Verification items for the finished model (mm, model axes). A direction names the side the tool comes from. Round coordinates to 2 decimals unless told otherwise and drop trailing zeros. Write each loop counter-clockwise with the first axis right and the second up, starting at its lowest first coordinate (ties: lowest second). Pieces come first, ordered by that corner, then holes. Notation, with made-up numbers: M -34.75,22.5 L 2.25,22.5 A9 ccw 2.25,33.5 Z; hole C -35,28.5 d2. An arc over 180 degrees is marked long. Use a Markdown table: item, result. Add a question column.
from build123d import *

# Parameters (mm, degrees)
BOSS_EXTRUDE1_DEPTH = 7.5
SKETCH2_R           = 3.5
CUT_EXTRUDE1_DEPTH  = 44.649720503
SKETCH6_R           = 3.5
CUT_EXTRUDE4_DEPTH  = 52.358372248
CUT_EXTRUDE5_DEPTH  = 1
CUT_EXTRUDE6_DEPTH  = 53.041544942
CUT_EXTRUDE7_DEPTH  = 1
CUT_EXTRUDE8_DEPTH  = 44.649720503
BOSS_EXTRUDE2_DEPTH = 22
BOSS_EXTRUDE3_START = -40
SKETCH12_W          = 15
SKETCH12_H          = 5
BOSS_EXTRUDE3_DEPTH = 40
CUT_EXTRUDE9_DEPTH  = 5


with BuildPart() as part:
    # Sketch1 → Boss-Extrude1 (new, symmetric)
    with BuildSketch(Plane(origin=(0, 0, 0), x_dir=(0, 0, -1), z_dir=(1, 0, 0))):
        Polygon((-15.91, -3), (-15.91, 3), (15.91, 3), (15.91, 37), (21.91, 37), (21.91, -3), align=None)
    extrude(amount=BOSS_EXTRUDE1_DEPTH, both=True)

    # Sketch2 → Cut-Extrude1 (cut, through all)
    with BuildSketch(Plane(origin=(0, 0, 0), x_dir=(1, 0, 0), z_dir=(0, 1, 0))):
        with Locations(Location((0, -9.41, 0), (0, 0, 90))):
            Circle(SKETCH2_R)
    extrude(amount=CUT_EXTRUDE1_DEPTH, mode=Mode.SUBTRACT)

    # Sketch6 → Cut-Extrude4 (cut, through all)
    with BuildSketch(Plane.XY.offset(-18.91)):
        with Locations((0, 30.5)):
            Circle(SKETCH6_R)
    extrude(amount=-CUT_EXTRUDE4_DEPTH, mode=Mode.SUBTRACT)

    # Sketch7 → Cut-Extrude5 (cut, symmetric)
    with BuildSketch(Plane.XY.offset(-18.91)):
        with BuildLine():
            Line((2.235057553, 16.161122159), (3.84429899, 30.054730114))
            ThreePointArc((3.84429899, 30.054730114), (3.863569405, 30.276994499), (3.87, 30.5))
            Line((3.87, 30.5), (3.87, 37))
            Line((3.87, 37), (-3.87, 37))
            Line((-3.87, 37), (-3.87, 30.5))
            ThreePointArc((-3.87, 30.5), (-3.863569405, 30.276994499), (-3.84429899, 30.054730114))
            Line((-3.84429899, 30.054730114), (-2.235057553, 16.161122159))
            ThreePointArc((-2.235057553, 16.161122159), (0, 14.17), (2.235057553, 16.161122159))
        make_face()
    extrude(amount=CUT_EXTRUDE5_DEPTH, both=True, mode=Mode.SUBTRACT)

    # Sketch8 → Cut-Extrude6 (cut, through all)
    with BuildSketch(Plane.XY.offset(-19.91)):
        with BuildLine():
            Line((3.87, 30.5), (3.87, 37))
            Line((3.87, 37), (-3.87, 37))
            Line((-3.87, 37), (-3.87, 30.5))
            ThreePointArc((-3.87, 30.5), (0, 26.63), (3.87, 30.5))
        make_face()
    extrude(amount=CUT_EXTRUDE6_DEPTH, mode=Mode.SUBTRACT)

    # Sketch9 → Cut-Extrude7 (cut, symmetric)
    with BuildSketch(Plane(origin=(0, 0, 0), x_dir=(1, 0, 0), z_dir=(0, 1, 0))):
        with BuildLine():
            Line((-3.87, -9.41), (-3.87, -15.91))
            Line((-3.87, -15.91), (3.87, -15.91))
            Line((3.87, -15.91), (3.87, -9.41))
            ThreePointArc((3.87, -9.41), (3.863569405, -9.186994499), (3.84429899, -8.964730114))
            Line((3.84429899, -8.964730114), (2.235057553, 4.928877841))
            ThreePointArc((2.235057553, 4.928877841), (0, 6.92), (-2.235057553, 4.928877841))
            Line((-2.235057553, 4.928877841), (-3.84429899, -8.964730114))
            ThreePointArc((-3.84429899, -8.964730114), (-3.863569405, -9.186994499), (-3.87, -9.41))
        make_face()
    extrude(amount=CUT_EXTRUDE7_DEPTH, both=True, mode=Mode.SUBTRACT)

    # Sketch10 → Cut-Extrude8 (cut, through all)
    with BuildSketch(Plane(origin=(0, 0, 0), x_dir=(1, 0, 0), z_dir=(0, 1, 0))):
        with BuildLine():
            Line((-3.87, -15.91), (3.87, -15.91))
            Line((3.87, -15.91), (3.87, -9.41))
            ThreePointArc((3.87, -9.41), (0, -5.54), (-3.87, -9.41))
            Line((-3.87, -9.41), (-3.87, -15.91))
        make_face()
    extrude(amount=-CUT_EXTRUDE8_DEPTH, mode=Mode.SUBTRACT)

    # Sketch11 → Boss-Extrude2 (add)
    with BuildSketch(Plane.XY.offset(15.91)):
        Polygon((-7.5, -3), (-3.87, -3), (-3.87, 1), (3.87, 1), (3.87, -3), (7.5, -3), (7.5, 3), (-7.5, 3), align=None)
    extrude(amount=BOSS_EXTRUDE2_DEPTH)

    # Sketch12 → Boss-Extrude3 (add)
    with BuildSketch(Plane.XZ.offset(3).offset(BOSS_EXTRUDE3_START)):
        with Locations((0, 35.41)):
            Rectangle(SKETCH12_W, SKETCH12_H)
    extrude(amount=BOSS_EXTRUDE3_DEPTH)

    # Sketch14 → Cut-Extrude9 (cut)
    with BuildSketch(Plane.XY.offset(37.91)):
        with BuildLine():
            Line((-2.625, 37), (-2.625, 30.5))
            ThreePointArc((-2.625, 30.5), (0, 27.875), (2.625, 30.5))
            Line((2.625, 30.5), (2.625, 37))
            Line((2.625, 37), (-2.625, 37))
        make_face()
    extrude(amount=-CUT_EXTRUDE9_DEPTH, mode=Mode.SUBTRACT)


solid = part.part
1. Cross-section at D-D on z = 18.5. Enter the section's corners in (x, y).
2. Depth check by flat-ended pin: pin 1 Ø10 at (y, z) = (27, -10) entering from -X; pin 2 Ø6 at (y, z) = (9.5, -14) entering from -X; pin 3 Ø7.5 at (x, z) = (-2, 12.5) entering from +Y. Enter the tip coordinate at first touch or a pass-through.
3. Scan lines: line 1 along Z through (x, y) = (1.25, 23); line 2 along Z through (x, y) = (-6.25, 22); line 3 along Z through (x, y) = (-3.5, 33). Record each from-to range of solid material in increasing order. Write a range as from..to.
4. Cross-section at B-B on x = 0. Enter the section's corners in (y, z) (3 decimals).
5. Cross-section at C-C on y = 21. Enter the section's corners in (x, z), plus the area to 3 significant figures.
6. Release check for a two-part mould opening along Z. For faces 1 (the flat face through (0, 17, 37.91)), 2 (the flat face through (-5, 37, 35)), 3 (the cylindrical face through (0.05, 0.01, -6.92)) record: +Z half, -Z half, draft (parallel to the pull), parting line (faces both ways), or undercut.
7. Cross-section at A-A on y = 12.5. Enter the section's corners in (x, z), plus the area to 3 significant figures.
8. Access from +Z, -Z, +X, -X, +Y, -Y to the whole of each face (thin tool, end or side, straight path). Record for faces 4 (the flat face through (-3.87, -1, 21)), 5 (the flat face through (3.87, 34, -18)), 6 (the flat face through (0, 1, 17)), 7 (the flat face through (0, 16, -15.91)), 8 (the flat face through (7.5, 2, 8)).
Answer:
| question | item | result |
|---|---|---|
| 1 | outline | M -7.5,-3 L -3.87,-3 L -3.87,1 L 3.87,1 L 3.87,-3 L 7.5,-3 L 7.5,3 L -7.5,3 Z |
| 2 | pin 1 | passes through |
| 2 | pin 2 | stops at x = -7.5 |
| 2 | pin 3 | stops at y = 3 |
| 3 | line 1 | z = -21.91..-19.91, -17.91..-15.91, 32.91..37.91 |
| 3 | line 2 | z = -21.91..-15.91, 32.91..37.91 |
| 3 | line 3 | z = -21.91..-19.91, 32.91..37.91 |
| 4 | outline | M -3,-21.91 L 27,-21.91 L 27,-19.91 L 14.17,-19.91 L 14.17,-17.91 L 26.63,-17.91 L 26.63,-15.91 L 3,-15.91 L 3,5.91 L 1,5.91 L 1,-6.92 L -1,-6.92 L -1,5.54 L -3,5.54 Z; M -3,32.91 L 1,32.91 L 1,12.91 L 3,12.91 L 3,32.91 L 27.875,32.91 L 27.875,37.91 L -3,37.91 Z; M 34,-21.91 L 37,-21.91 L 37,-19.91 L 34,-19.91 Z |
| 5 | outline | M -7.5,-21.91 L 7.5,-21.91 L 7.5,-15.91 L -7.5,-15.91 Z; M -7.5,32.91 L 7.5,32.91 L 7.5,37.91 L -7.5,37.91 Z; hole M -2.8,-19.91 L 2.8,-19.91 L 2.8,-17.91 L -2.8,-17.91 Z |
| 5 | area | 154 mm^2 |
| 6 | face 1 | +Z half |
| 6 | face 2 | draft |
| 6 | face 3 | undercut |
| 7 | outline | M -7.5,-21.91 L 7.5,-21.91 L 7.5,-15.91 L -7.5,-15.91 Z; M -7.5,32.91 L 7.5,32.91 L 7.5,37.91 L -7.5,37.91 Z |
| 7 | area | 165 mm^2 |
| 8 | face 4 | -Y |
| 8 | face 5 | +Y |
| 8 | face 6 | none |
| 8 | face 7 | +X, -X, +Y |
| 8 | face 8 | +Z, -Z, +X, +Y, -Y |
